For this review, take the finished solid that the model builds, in its own axes (mm). A direction names the side the tool comes from. Round coordinates to 2 decimals unless told otherwise and drop trailing zeros. Order: outer loops, then holes, each group sorted by start corner. A loop starts at its lowest first (then second) coordinate and runs counter-clockwise, first axis right, second up. Notation, with made-up numbers: M 53.5,-19 L 71.5,-19 A21 cw 71.5,11 Z; hole C -14.75,76.5 d11. An arc over 180 degrees is marked long. Put each result on its own line as item: value.
Autodesk Inventor part; units mm, degrees
ref_plane "YZ Plane" through (0, 0, 0) normal (1, 0, 0) x (0, 1, 0)
ref_plane "XZ Plane" through (0, 0, 0) normal (0, 1, 0) x (-1, 0, 0)
ref_plane "XY Plane" through (0, 0, 0) normal (0, 0, 1) x (1, 0, 0)
sketch "Sketch1" plane through (0, 0, 0) normal (0, 1, 0) x (-1, 0, 0)
  line L0 (-20.25, 15) -> (20.25, 15)
  line L1 (20.25, 15) -> (20.25, -15)
  line L2 (20.25, -15) -> (-20.25, -15)
  line L3 (-20.25, -15) -> (-20.25, 15)
  line L4 (-20.25, 15) -> (20.25, -15) construction
  line L5 (20.25, 15) -> (-20.25, -15) construction
  point P0 (0, 0)
  dimension "d0" = 30
  dimension "d1" = 40.5
extrude "Plate1" add sketch "Sketch1" along normal blind 1.5
sketch "Sketch2" plane through (21.75, 0, -15) normal (-1, 0, 0) x (0, -1, 0)
  line L0 (0, 30) -> (0, 0)
  line L1 (0, 0) -> (-30, 0)
  line L2 (-30, 0) -> (-30, 30)
  line L3 (-30, 30) -> (0, 30)
edge flange "Flange1" height 30 angle 90 thickness 1.5 bend radius 0.31 thickness toward (-1, 0, 0) relief tear relief width 1.5 relief depth 0.75 corner gap 0.31 corner form 0 edges at (20.25, 1.5, 0) (-20.25, 1.5, 0) wall of the first edge with corners at (21.75, 0, 15) (21.75, 0, -15) (21.75, 30, -15) (21.75, 30, 15)
bend "Bend1"
corner "Corner1"
sketch "Sketch3" plane through (-21.75, 30, -15) normal (-1, 0, 0) x (0, 0, 1)
  point P0 (15, -30)
equation "\"d2\" = Thickness"
equation "\"d3\" = BendReliefWidth"
equation "\"d4\" = BendReliefDepth"
equation "\"d5\" = MinimumRemnant"
equation "\"d6\" = TransitionRadius"
equation "\"d9\" = BendRadius"
equation "\"d10\" = CornerReliefSize"
equation "\"d11\" = GapSize"
equation "\"d12\" = JacobiRadiusSize"
equation "\"BendReliefWidth\" = Thickness"
equation "\"BendReliefDepth\" = 0.5 * Thickness"
equation "\"CornerReliefSize\" = 4 * Thickness"
equation "\"MinimumRemnant\" = 2 * Thickness"
equation "\"TransitionRadius\" = BendRadius"
equation "\"JacobiRadiusSize\" = BendRadius"
equation "\"GapSize\" = Thickness"
properties part number "hurseong" material "Aluminum 6061-AHC"
(1) For faces 5 (the face through (-21.23, 0.54, 0.21)), 6 (the face through (-20.25, 16, 0)), list the 3-axis set-ups (+Z, -Z, +X, -X, +Y, -Y) from which the entire face can be reached by the end or side of a thin tool; tool diameter is ignored.
A:
face 5: +Z, -Z, -X, -Y
face 6: +Z, -Z, +Y
(2) To check wall thickness, follow L1, parallel to X at y = 11.75, z = -9.25; L2, parallel to Y at x = 14, z = 12.5. State the ranges of each line that lie inside material, in increasing order.
A:
L1: x = -21.75 to -20.25, 20.25 to 21.75
L2: y = 0 to 1.5
(3) Draft analysis for pull direction X (two halves, no side actions). For faces 1 (the face through (-21, 30, 0)), 2 (the face through (21.75, 16, 0)), 3 (the face through (20.25, 16, 0)), 4 (the face through (0, 1.5, 0)), state which applies: released by +X, released by -X, zero draft, split by the parting line, or undercut.
A:
face 1: zero draft
face 2: released by +X
face 3: undercut
face 4: undercut
(4) Add section C-C on x = -9. Give the boundary of the cut face in (y, z).
A:
outline: M 0,-15 L 1.5,-15 L 1.5,15 L 0,15 Z
(5) Add section A-A on y = 22. Give the boundary of the cut face in (x, z), then the cut area to 3 significant figures.
A:
outline: M -21.75,-15 L -20.25,-15 L -20.25,15 L -21.75,15 Z; M 20.25,-15 L 21.75,-15 L 21.75,15 L 20.25,15 Z
area: 90.0 mm2
(6) Add section B-B on z = -8. Give the boundary of the cut face in (x, y).
A:
outline: M -21.75,1.81 A1.81 ccw -19.94,0 L 19.94,0 A1.81 ccw 21.75,1.81 L 21.75,30 L 20.25,30 L 20.25,1.81 A0.31 cw 19.94,1.5 L -19.94,1.5 A0.31 cw -20.25,1.81 L -20.25,30 L -21.75,30 Z
(7) Insertion check: pin 1 Ø15 at (x, z) = (1, -7) entering from +Y. The pin has a flat end and moves straight along its axis. Give the tip position at first contact, or say it passes through.
A:
pin 1: stops at y = 1.5
